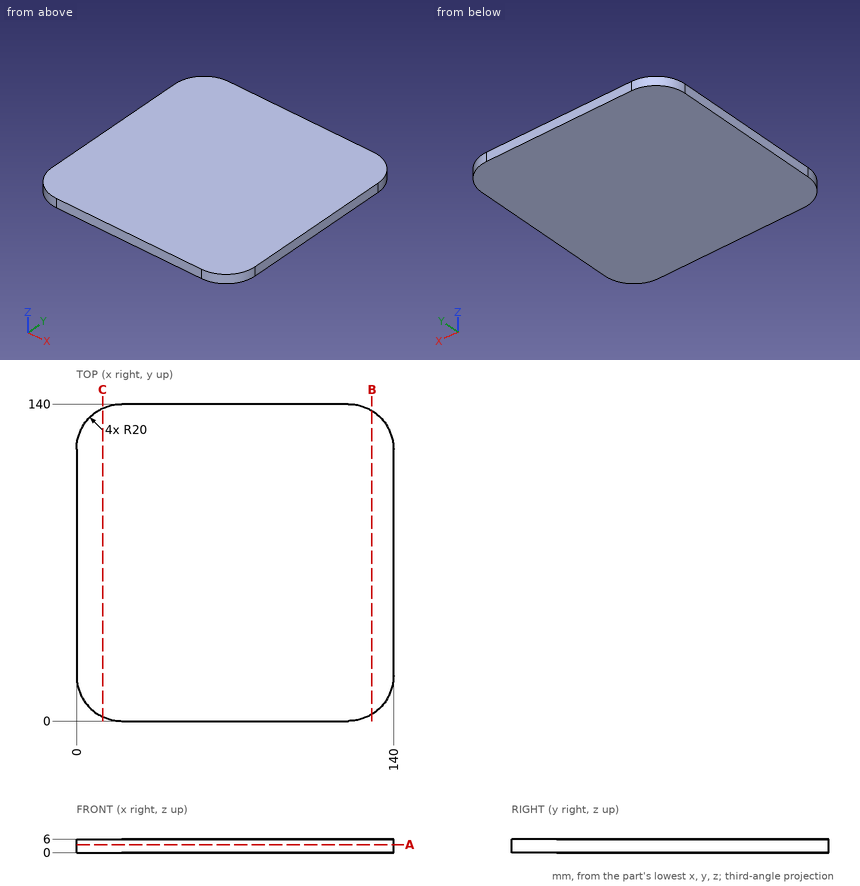
Input: dimensioned drawing with shaded views. Units: mm. Origin: part minimum x, y, z. Coordinates: 2 decimals unless noted, no trailing zeros. Write each loop counter-clockwise with the first axis right and the second up, starting at its lowest first coordinate (ties: lowest second). Pieces come first, ordered by that corner, then holes. Notation, with made-up numbers: M 42.25,22.5 L 93.25,22.5 A7 ccw 93.25,29.5 Z; hole C 13,65.5 d7. An arc over 180 degrees is marked long. Use one line per item in the form item = value.
Q1. Material intervals for probe 1 along X at (y, z) = (121, 3.95); probe 2 along X at (y, z) = (8, 1.85); probe 3 along Y at (x, z) = (12, 0.9), sorted ascending. Write a range as from..to.
Answer below:
probe_1 = 0.03..139.97
probe_2 = 4..136
probe_3 = 1.67..138.33
Q2. Section B-B (x = 130.5). Return loops of the section in (y, z).
Answer below:
outline = M 2.98,0 L 137.02,0 L 137.02,6 L 2.98,6 Z
Q3. Section C-C (x = 11.5). Return loops of the section in (y, z), plus the area to 3 significant figures.
Answer below:
outline = M 1.9,0 L 138.1,0 L 138.1,6 L 1.9,6 Z
area = 817 mm²
Q4. Section A-A (z = 3.5). Return loops of the section in (x, y), plus the area to 3 significant figures.
Answer below:
outline = M 0,20 A20 ccw 20,0 L 120,0 A20 ccw 140,20 L 140,120 A20 ccw 120,140 L 20,140 A20 ccw 0,120 Z
area = 19,300 mm²
